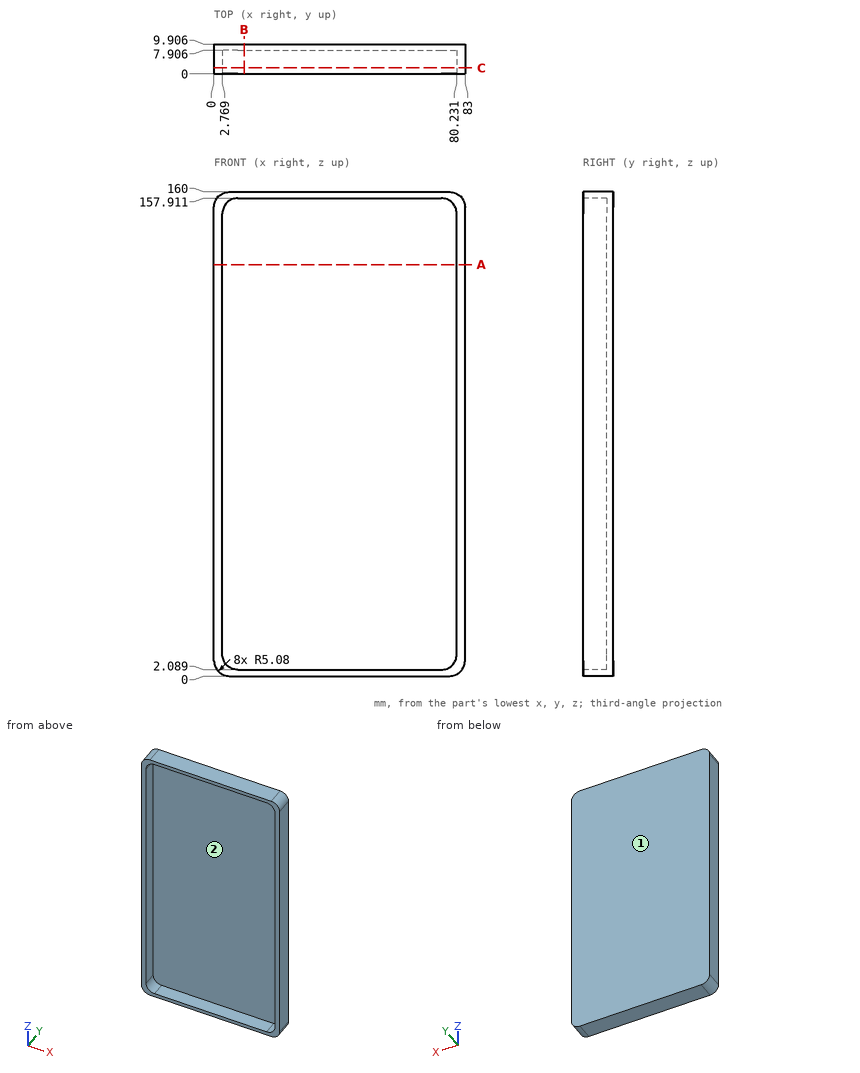
Geometry check sheet. Reference: drawing and pictorial views, mm from the part's lowest x, y, z. Give positions to 0.01 mm unless a question says otherwise; leave off trailing zeros. Loops run counter-clockwise (first coordinate to the right, second up) from the corner with the lowest first, then second, coordinate; pieces in that order, holes last. Notation, with made-up numbers: (25.25, -15.5) - (63.25, -15.5) arc R22 ccw to (63.25, -5.5) - close; hole circle Ø8 at (43.5, 51.25). An arc over 180 degrees is marked (long way). Use CSV: the item, a comma, the result in double quotes. Start each with the question number.
Q1. Scan lines: probe 1 along Z at (x, y) = (27, 1.75); probe 2 along X at (y, z) = (2.25, 93); probe 3 along Y at (x, z) = (60.5, 140.5) (1 decimal). Record each from-to range of solid material in increasing order. Write a range as from..to.
Q2. Section check A-A, the plane z = 136. Record the cut outline in (x, y) (1 decimal), and give its area (3 significant figures).
Q3. Section check B-B, the plane x = 10. Record the cut outline in (y, z) (1 decimal).
Q4. Release check for a two-part mould opening along Z. For the marked faces 1 and 2 record: +Z half, -Z half, draft (parallel to the pull), parting line (faces both ways), or undercut.
Q5. Section check C-C, the plane y = 2. Record the cut outline in (x, z).
Q6. Go/stop test with a flat-tipped pin: pin 1 Ø6 at (x, z) = (70, 22.5) entering from -Y. Record where the tip stops, or that it passes through.
Findings below:
1,probe 1,"z = 0..2.09, 157.91..160"
1,probe 2,"x = 0..2.77, 80.23..83"
1,probe 3,"y = 7.9..9.9"
2,outline,"(0, 0) - (2.8, 0) - (2.8, 7.9) - (80.2, 7.9) - (80.2, 0) - (83, 0) - (83, 9.9) - (0, 9.9) - close"
2,area,"210 mm^2"
3,outline,"(0, 0) - (9.9, 0) - (9.9, 160) - (0, 160) - (0, 157.9) - (7.9, 157.9) - (7.9, 2.1) - (0, 2.1) - close"
4,face 1,"draft"
4,face 2,"undercut"
5,outline,"(0, 5.08) arc R5.08 ccw to (5.08, 0) - (77.92, 0) arc R5.08 ccw to (83, 5.08) - (83, 154.92) arc R5.08 ccw to (77.92, 160) - (5.08, 160) arc R5.08 ccw to (0, 154.92) - close; hole (2.77, 7.17) arc R5.08 ccw to (7.85, 2.09) - (75.15, 2.09) arc R5.08 ccw to (80.23, 7.17) - (80.23, 152.83) arc R5.08 ccw to (75.15, 157.91) - (7.85, 157.91) arc R5.08 ccw to (2.77, 152.83) - close"
6,pin 1,"stops at y = 7.91"
